Read the model definition and answer for the solid it produces. Units are mm, in the model's axes. A direction names the side the tool comes from. Give positions to 0.01 mm unless a question says otherwise; leave off trailing zeros. Loops run counter-clockwise (first coordinate to the right, second up) from the corner with the lowest first, then second, coordinate; pieces in that order, holes last. Notation, with made-up numbers: (-25, 63.5) - (11, 63.5) arc R19 ccw to (11, 92.5) - close; hole circle Ø6 at (26, 38). An arc over 180 degrees is marked (long way). Write item = value, one per line.
```python
from build123d import *

# Parameters (mm, degrees)
SKETCH1_W           = 350
SKETCH1_H           = 300
SKETCH1_R           = 60
BOSS_EXTRUDE1_DEPTH = 10
SKETCH2_W           = 400
SKETCH2_H           = 300
BOSS_EXTRUDE2_DEPTH = 10
SKETCH3_W           = 350
SKETCH3_H           = 400
BOSS_EXTRUDE3_DEPTH = 10


with BuildPart() as part:
    # Sketch1 → Boss-Extrude1 (new body)
    with BuildSketch(Plane.XY):
        Rectangle(SKETCH1_W, SKETCH1_H)
        with Locations((0, -2.864034897)):
            Circle(SKETCH1_R, mode=Mode.SUBTRACT)
    extrude(amount=BOSS_EXTRUDE1_DEPTH)

    # Sketch2 → Boss-Extrude2 (add)
    with BuildSketch(Plane.ZY.offset(175)):
        with Locations((200, 0)):
            Rectangle(SKETCH2_W, SKETCH2_H)
    boss_extrude2 = extrude(amount=-BOSS_EXTRUDE2_DEPTH)

    # Mirror1: Boss-Extrude2 across plane
    add(boss_extrude2.mirror(Plane(origin=(0, 0, 0), x_dir=(0, 0, 1), z_dir=(1, 0, 0))))

    # Sketch3 → Boss-Extrude3 (add)
    with BuildSketch(Plane.XZ.offset(150)):
        with Locations((0, 200)):
            Rectangle(SKETCH3_W, SKETCH3_H)
    boss_extrude3 = extrude(amount=-BOSS_EXTRUDE3_DEPTH)

    # Mirror2: Boss-Extrude3 across plane
    add(boss_extrude3.mirror(Plane.ZX))


solid = part.part
```
1) Find the intervals of material crossed by probe 1 along Y at (x, z) = (37, 87.5); probe 2 along X at (y, z) = (-34.5, 192.5); probe 3 along Y at (x, z) = (0, 4.5), in increasing order.
Output:
probe_1 = -150 to -140, 140 to 150
probe_2 = -175 to -165, 165 to 175
probe_3 = -150 to -62.86, 57.14 to 150
2) The mould has two halves that part along Y. Classify faces 1 (the face through (-2, 150, 197)), 2 (the face through (-1, -145, 400)), 3 (the face through (-13.007, -61.437, 4.93)): pulls with the +Y half, pulls with the -Y half, needs draft (parallel to the pull), parting line crosses it, or undercut.
Output:
face_1 = pulls with the +Y half
face_2 = needs draft
face_3 = undercut
3) A cutting plane is placed at B-B on z = 100. Determine the outline of the cut face in (x, y), then the cut area to 3 significant figures.
Output:
outline = (-175, -150) - (175, -150) - (175, 150) - (-175, 150) - close; hole (-165, -140) - (165, -140) - (165, 140) - (-165, 140) - close
area = 12,600 mm²
4) A cutting plane is placed at D-D on x = -91. Determine the outline of the cut face in (y, z).
Output:
outline = (-150, 0) - (150, 0) - (150, 400) - (140, 400) - (140, 10) - (-140, 10) - (-140, 400) - (-150, 400) - close
5) A tool of negligible diameter and unlimited length cuts with its end or side. For faces 4 (the face through (-175, -2, 197)), 5 (the face through (-2, -140, 208)), from which of +Z, -Z, +X, -X, +Y, -Y can it reach the whole face along a straight path? Write none if from no direction.
Output:
face_4 = +Z, -Z, -X, +Y, -Y
face_5 = +Z
6) A cutting plane is placed at C-C on y = -89.5. Determine the outline of the cut face in (x, z).
Output:
outline = (-175, 0) - (175, 0) - (175, 400) - (165, 400) - (165, 10) - (-165, 10) - (-165, 400) - (-175, 400) - close
7) A cutting plane is placed at A-A on x = 0. Determine the outline of the cut face in (y, z), then the cut area to 3 significant figures.
Output:
outline = (-150, 0) - (-62.86, 0) - (-62.86, 10) - (-140, 10) - (-140, 400) - (-150, 400) - close; (57.14, 0) - (150, 0) - (150, 400) - (140, 400) - (140, 10) - (57.14, 10) - close
area = 9,600 mm²
